```python
from build123d import *

# Parameters (mm, degrees)
SKETCH_2_R               = 6
SKETCH_2_R_2             = 2.5
EXTRUDE_1_DEPTH          = 4
EXTRUDE_2_DEPTH          = 0.2
SKETCH_2_5_R             = 6
SKETCH_2_5_R_2           = 2.5
EXTRUDE_6_DEPTH          = 2
PATTERN_CIRCULAR_1_COUNT = 6


with BuildPart() as part:
    # 草图2 → 凸台-拉伸1 (new body)
    with BuildSketch(Plane.XY):
        Circle(SKETCH_2_R)
        Circle(SKETCH_2_R_2, mode=Mode.SUBTRACT)
    extrude(amount=EXTRUDE_1_DEPTH)

    # 草图6 → 凸台-拉伸2 (add, symmetric)
    with BuildSketch(Plane(origin=(0, 0, 0), x_dir=(0.9659258262890681, 0, -0.2588190451025218), z_dir=(0.2588190451025218, 0, 0.9659258262890681))):
        with BuildLine():
            Line((4, 2.970800909), (6.665063509, 7.586826313))
            ThreePointArc((6.665063509, 7.586826313), (6.914814566, 8.1897787), (7, 8.836826313))
            Line((7, 8.836826313), (7, 32))
            ThreePointArc((7, 32), (6.121320344, 34.121320344), (4, 35))
            Line((4, 35), (2.519223828, 35))
            ThreePointArc((2.519223828, 35), (-0.267681994, 34.186020016), (-2.178368771, 32))
            add(Edge.make_bspline(
                [(-2.178368771, 32), (-6.131576328, 18.074358524), (0.381779744, 5.817884597)],
                knots=[0, 0, 0, 1, 1, 1], degree=2))
            add(Edge.make_bspline(
                [(4, 2.970800909), (2.776948837, 5.192610395), (0.381779744, 5.817884597)],
                knots=[5.230377445, 5.230377445, 5.230377445, 6.036173694, 6.036173694, 6.036173694], degree=2, weights=[1, 0.919928545, 1]))
        make_face()
    extrude_2 = extrude(amount=EXTRUDE_2_DEPTH, both=True)

    # 草图2<5> → 凸台-拉伸6 (add, symmetric)
    with BuildSketch(Plane.XY):
        Circle(SKETCH_2_5_R)
        Circle(SKETCH_2_5_R_2, mode=Mode.SUBTRACT)
    extrude(amount=EXTRUDE_6_DEPTH, both=True)

    # 阵列(圆周)1: 凸台-拉伸2 ×6 about axis
    pattern_circular_1_axis = Axis((0, 0, 4), (0, 0, -1))
    for i in range(1, PATTERN_CIRCULAR_1_COUNT):
        add(extrude_2.rotate(pattern_circular_1_axis, i * 360 / PATTERN_CIRCULAR_1_COUNT))


solid = part.part
```
Check sheet for the modelled part. Datum: model origin and axes. Units: mm. A direction names the side the tool comes from. Coordinates: 2 decimals unless noted, no trailing zeros. Write item = value, one per line. Start each with the question number.
1. Thickness scan on probe 1 along Y at (x, z) = (0, 2.75); probe 2 along Y at (x, z) = (0, 0); probe 3 along Z at (x, y) = (0.5, -25). Record the ranges inside material, lowest first.
2. Go/stop test with flat-tipped pins: pin 1 (5 mm diameter, centred on x = 19.5, y = -5.5, fed in from -Z); pin 2 (9.5 mm diameter, centred on x = 1, y = -1, fed in from -Z); pin 3 (1 mm diameter, centred on y = -15, z = 1, fed in from +X). Record where each tip stops, or that it passes through.
3. Mould release check, pull along Y, two halves, no side actions. Record for faces 4 (the flat face through (-17.972, -8.295, -0.276)), 5 (the cylindrical face through (26.56, -22.19, -1.59)), 6 (the flat face through (-2.28, 7.58, -1.45)): pulls with the +Y half, pulls with the -Y half, needs draft (parallel to the pull), parting line crosses it, or undercut.
4. Tool access check on faces 1 (the flat face through (-16.169, 11.416, -0.276)), 2 (the flat face through (-1.802, -19.711, -0.276)), 3 (the flat face through (-16.25, 11.34, -0.66)). Record the directions out of +Z, -Z, +X, -X, +Y, -Y that give a thin tool (end or side, any length) a straight path to the whole face; none if there is none.
The answers:
q1.probe_1 = -6 to -2.5, 2.5 to 6
q1.probe_2 = -34.35 to -6.56, -6 to -2.5, 2.5 to 6, 6.56 to 34.35
q1.probe_3 = -0.07 to 0.34
q2.pin_1 = 0.46
q2.pin_2 = -2
q2.pin_3 = 29.33
q3.face_4 = undercut
q3.face_5 = pulls with the -Y half
q3.face_6 = pulls with the +Y half
q4.face_1 = +Z, +Y
q4.face_2 = +Z, -Y
q4.face_3 = -Z, -X
